from build123d import *

# Parameters (mm, degrees)
F0_W     = 29
F0_H     = 23
F0_W_2   = 27
F0_H_2   = 21
F1_DEPTH = 10
F2_DEPTH = 9
F3_W     = 1.23707
F3_H     = 11.001679
F4_DEPTH = 9
F5_W     = 8.081423
F5_H     = 0.370867
F6_DEPTH = 5


with BuildPart() as f1:
    # F0 (on Front) → F1 (new body)
    with BuildSketch(Plane.XZ):
        Rectangle(F0_W, F0_H)
        Rectangle(F0_W_2, F0_H_2, mode=Mode.SUBTRACT)
        Rectangle(F0_W_2, F0_H_2)
    extrude(amount=F1_DEPTH)

    # F0 (on Front) → F2 (cut)
    with BuildSketch(Plane.XZ):
        Rectangle(F0_W_2, F0_H_2)
    extrude(amount=F2_DEPTH, mode=Mode.SUBTRACT)

    # F3 (on face) → F4 (cut)
    with BuildSketch(Plane.XZ):
        with Locations((14.021569, 5.029028)):
            Rectangle(F3_W, F3_H)
    extrude(amount=F4_DEPTH, mode=Mode.SUBTRACT)

    # F5 (on face) → F6 (cut)
    with BuildSketch(Plane.XZ):
        Polygon((-10.967096, 11.561035), (-10.967096, 11.5), (-2.885673, 11.5), (-2.885673, 11.855262), (-10.967096, 11.855262), align=None)
        with Locations((-6.926384, 10.314566)):
            Rectangle(F5_W, F5_H)
        Polygon((-10.967096, 11.5), (-10.967096, 10.521435), (-10.967096, 10.5), (-2.885673, 10.5), (-2.885673, 11.5), align=None)
    extrude(amount=F6_DEPTH, mode=Mode.SUBTRACT)


solid = f1.part
Verification items for the finished model (mm, model axes). A direction names the side the tool comes from. Coordinates: 2 decimals unless noted, no trailing zeros. Order: outer loops, then holes, each group sorted by start corner. A loop starts at its lowest first (then second) coordinate and runs counter-clockwise, first axis right, second up. Notation, with made-up numbers: M 55.25,-32 L 65.25,-32 A11 ccw 65.25,-25 Z; hole C 45,37 d7. An arc over 180 degrees is marked long. One line per item, written item: value. Start each with the question number.
Item 1: Depth check by flat-ended pin: P1, Ø0.5, axis at x = -5.5, z = 11, coming from the +Y side; P2, Ø2, axis at x = 1.5, z = -4, coming from the +Y side. Enter the tip coordinate at first touch or a pass-through.
Item 2: Access from +Z, -Z, +X, -X, +Y, -Y to the whole of each face (thin tool, end or side, straight path). Record for faces 4 (the flat face through (0, -4, -10.5)), 5 (the flat face through (14, -4, 10.53)), 6 (the flat face through (-10.967, -2, 11)).
Item 3: Sectioned sample at D-D on z = -1.5. Record the cut outline in (x, y), then the cut area to 3 significant figures.
Item 4: Thickness scan on probe 1 along X at (y, z) = (-2, -1.25); probe 2 along Z at (x, y) = (7.75, -2); probe 3 along Y at (x, z) = (0.5, -1.25). Record the ranges inside material, lowest first.
Item 5: Mould release check, pull along Z, two halves, no side actions. Record for faces 1 (the flat face through (-3, 0, -11)), 2 (the flat face through (0, -5, 11.5)), 3 (the flat face through (-13.5, -4, 0)): pulls with the +Z half, pulls with the -Z half, needs draft (parallel to the pull), parting line crosses it, or undercut.
Item 6: Sectioned sample at B-B on x = -12.5. Record the cut outline in (y, z), then the cut area to 3 significant figures.
Calculated:
1. P1: y = -5
1. P2: y = -9
2. face 4: +Y
2. face 5: +X, +Y
2. face 6: +Z, +Y
3. outline: M -14.5,-10 L 14.5,-10 L 14.5,0 L 13.5,0 L 13.5,-9 L -13.5,-9 L -13.5,0 L -14.5,0 Z
3. area: 47.0 mm^2
4. probe 1: -14.5 to -13.5, 13.5 to 14.5
4. probe 2: -11.5 to -10.5, 10.5 to 11.5
4. probe 3: -10 to -9
5. face 1: needs draft
5. face 2: pulls with the +Z half
5. face 3: undercut
6. outline: M -10,-11.5 L 0,-11.5 L 0,-10.5 L -9,-10.5 L -9,10.5 L 0,10.5 L 0,11.5 L -10,11.5 Z
6. area: 41.0 mm^2
